```python
from build123d import *

# Parameters (mm, degrees)
SKETCH_1_W          = 5
SKETCH_1_H          = 2.75
EXTRUDE_1_DEPTH     = 2.75
SKETCH_2_W          = 7
SKETCH_2_H          = 10
CUT_EXTRUDE_1_DEPTH = 10


with BuildPart() as part:
    # 草图1 → 凸台-拉伸1 (new body)
    with BuildSketch(Plane.XY):
        Polygon((95, 100), (100, 100), (100, 102.75), (95, 102.75), (95, 102.449578136), align=None)
        Polygon((3, 3), (3, 0), (97, 0), (97, 3), (100, 3), (100, 100), (95, 100), (5, 100), (0, 100), (0, 3), align=None)
        with Locations((2.5, 101.375)):
            Rectangle(SKETCH_1_W, SKETCH_1_H)
        Polygon((0, 0), (0, -30), (10, -30), (30, -30), (30, -27), (50, -27), (70, -27), (70, -30), (90, -30), (100, -30), (100, 0), (97, 0), (3, 0), align=None)
        Polygon((30, -30), (10, -30), (10, -33), (90, -33), (90, -30), (70, -30), (50, -30), align=None)
    extrude(amount=EXTRUDE_1_DEPTH)

    # 草图2 → 切除-拉伸1 (cut)
    with BuildSketch(Plane.XY.offset(2.75)):
        with Locations((13.5, -20)):
            Rectangle(SKETCH_2_W, SKETCH_2_H)
    extrude(amount=-CUT_EXTRUDE_1_DEPTH, mode=Mode.SUBTRACT)


solid = part.part
```
Geometry check sheet. Reference: the model listing, model coordinates, mm. A direction names the side the tool comes from. Coordinates: 2 decimals unless noted, no trailing zeros. Write each loop counter-clockwise with the first axis right and the second up, starting at its lowest first coordinate (ties: lowest second). Pieces come first, ordered by that corner, then holes. Notation, with made-up numbers: M -11.5,-21.75 L 34.5,-21.75 A20 cw 34.5,15.25 Z; hole C -29.75,79 d5. An arc over 180 degrees is marked long. One line per item, written item: value. Start each with the question number.
(1) Sectioned sample at C-C, the plane z = 2.3. Enter the section's corners in (x, y), and give its area (3 significant figures).
(2) Tool access check on faces 1 (the face through (50, -30, 1)), 2 (the face through (97, 1, 1)), 3 (the face through (3, 2, 1)). Record the directions out of +Z, -Z, +X, -X, +Y, -Y that give a thin tool (end or side, any length) a straight path to the whole face; none if there is none.
(3) Depth check by flat-ended pin: pin 1 (0.8 mm diameter, centred on x = 98, z = 0.5, fed in from -Y); pin 2 (1.5 mm diameter, centred on x = 28, z = 0.5, fed in from +Y); pin 3 (0.8 mm diameter, centred on y = -31, z = 1, fed in from -X). Enter the tip coordinate at first touch or a pass-through.
(4) Sectioned sample at D-D, the plane x = 84. Enter the section's corners in (y, z).
(5) Release check for a two-part mould opening along Y. For faces 4 (the face through (90, -32, 1)), 5 (the face through (13, -25, 1)), 6 (the face through (51, 100, 1)) record: released by +Y, released by -Y, zero draft, split by the parting line, or undercut.
(6) Scan lines: line 1 along Y through (x, z) = (61, 2.6); line 2 along X through (y, z) = (-21, 0.55); line 3 along Y through (x, z) = (29.5, 1.1). Record each from-to range of solid material in increasing order. Write a range as [from, to].
(7) Sectioned sample at A-A, the plane x = 11.5. Enter the section's corners in (y, z), and give its area (3 significant figures).
(8) Sectioned sample at B-B, the plane y = -17. Enter the section's corners in (x, z), and give its area (3 significant figures).
Filled sheet:
1. outline: M 0,-30 L 10,-30 L 10,-33 L 90,-33 L 90,-30 L 100,-30 L 100,0 L 97,0 L 97,3 L 100,3 L 100,102.75 L 95,102.75 L 95,100 L 5,100 L 5,102.75 L 0,102.75 L 0,3 L 3,3 L 3,0 L 0,0 Z; hole M 10,-25 L 17,-25 L 17,-15 L 10,-15 Z; hole M 30,-30 L 70,-30 L 70,-27 L 30,-27 Z
1. area: 13,100 mm²
2. face 1: +Z, -Z
2. face 2: +Z, -Z, +X
2. face 3: +Z, -Z, -X
3. pin 1: y = -30
3. pin 2: y = 100
3. pin 3: x = 10
4. outline: M -33,0 L 100,0 L 100,2.75 L -33,2.75 Z
5. face 4: zero draft
5. face 5: undercut
5. face 6: released by +Y
6. line 1: [-33, -30], [-27, 100]
6. line 2: [0, 10], [17, 100]
6. line 3: [-33, 100]
7. outline: M -33,0 L -25,0 L -25,2.75 L -33,2.75 Z; M -15,0 L 100,0 L 100,2.75 L -15,2.75 Z
7. area: 338 mm²
8. outline: M 0,0 L 10,0 L 10,2.75 L 0,2.75 Z; M 17,0 L 100,0 L 100,2.75 L 17,2.75 Z
8. area: 256 mm²
